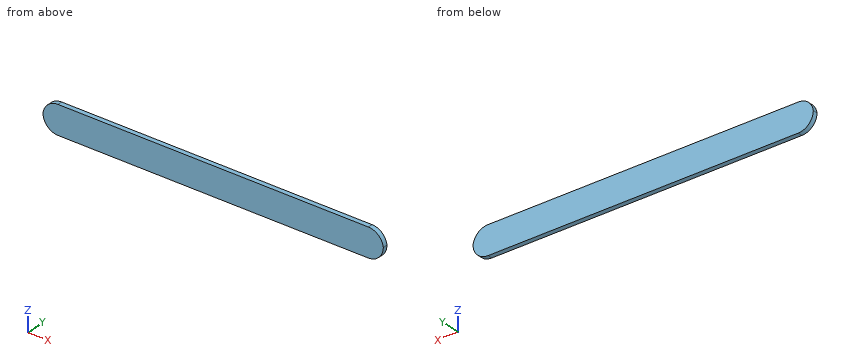
```python
from build123d import *

# Parameters (mm, degrees)
F0_W        = 114.3
F0_H        = 9.525
F1_DEPTH    = 1.5875
F2_R        = 5.08
F3_T1_DEPTH = 26.7882812379
F4_R        = 5.08
F5_T1_DEPTH = 26.7882812379


# Not quite as in the source:
# - a fillet or chamfer that OpenCascade refuses, or shapes differently, is made with other operations: its cross-section is extruded or revolved along the edge and cut away or added


with BuildPart() as f1:
    # F0 (on Front) → F1 (new body)
    with BuildSketch(Plane.XZ):
        with Locations((-7.7723998189, 23.2028993189)):
            Rectangle(F0_W, F0_H)
    extrude(amount=F1_DEPTH)

    # F2
    f2_edges = [f1.edges().sort_by_distance(p)[0] for p in [
        (-64.9224, -0.79375, 18.440399),
    ]]
    fillet(f2_edges, radius=F2_R)

    # F3: fillet of radius 5.08 on 1 edges, made by hand

    # F3_s2 → F3_t1 (cut)
    with BuildSketch(Plane.XZ.offset(-12.6003906189)):
        with BuildLine():
            ThreePointArc((-64.9223998189, 23.5203993189), (-63.2423477364, 26.6953993189), (-59.8822435713, 27.9653993189))
            Line((-59.8822435713, 27.9653993189), (-64.9223998189, 27.9653993189))
            Line((-64.9223998189, 27.9653993189), (-64.9223998189, 23.5203993189))
        make_face()
    extrude(amount=F3_T1_DEPTH, mode=Mode.SUBTRACT)

    # F4
    f4_edges = [f1.edges().sort_by_distance(p)[0] for p in [
        (49.3776, -0.79375, 18.440399),
    ]]
    fillet(f4_edges, radius=F4_R)

    # F5: fillet of radius 5.08 on 1 edges, made by hand

    # F5_s2 → F5_t1 (cut)
    with BuildSketch(Plane.XZ.offset(-12.6003906189)):
        with BuildLine():
            ThreePointArc((49.3776001811, 23.5203993189), (47.6975480986, 26.6953993189), (44.3374439335, 27.9653993189))
            Line((44.3374439335, 27.9653993189), (49.3776001811, 27.9653993189))
            Line((49.3776001811, 27.9653993189), (49.3776001811, 23.5203993189))
        make_face()
    extrude(amount=F5_T1_DEPTH, mode=Mode.SUBTRACT)


solid = f1.part
```
Here's how the part is built. I have some questions about the finished solid (model axes, mm). Round coordinates to 2 decimals unless told otherwise and drop trailing zeros. Loops run counter-clockwise (first coordinate to the right, second up) from the corner with the lowest first, then second, coordinate; pieces in that order, holes last. Notation, with made-up numbers: (66, 54) -> (72, 54) arc R16 ccw to (72, 74) -> close; hole circle Ø10 at (-25.75, -39.75). An arc over 180 degrees is marked (long way). Answer as CSV lines item,"result". Start each with the question number.
1. I need wall thicknesses on probe 1 along X at (y, z) = (-0.3, 19.5); probe 2 along X at (y, z) = (-0.25, 22.5). Which ranges of each line are inside material? Lowest first, please. Write a range as from..to.
2. Imagine slicing it at A-A on y = -0.4. Write out the boundary of the cut face in (x, z), plus the area to 3 significant figures.
3. Imagine slicing it at B-B on z = 20.5. Write out the boundary of the cut face in (x, y), plus the area to 3 significant figures.
Solution:
1,probe 1,"-62.95..47.4"
1,probe 2,"-64.82..49.27"
2,outline,"(-64.92, 23.52) arc R5.08 ccw to (-59.84, 18.44) -> (44.3, 18.44) arc R5.08 ccw to (49.38, 23.52) arc R5.08 ccw to (44.34, 27.97) -> (-59.88, 27.97) arc R5.08 ccw to start"
2,area,"1,070 mm²"
3,outline,"(-63.93, -1.59) -> (48.38, -1.59) -> (48.38, 0) -> (-63.93, 0) -> close"
3,area,"178 mm²"
